```python
from build123d import *

# Parameters (mm, degrees)
F0_W     = 12.8
F0_H     = 6.4
F1_DEPTH = 1
F0_W_2   = 20
F0_H_2   = 12
F2_DEPTH = 160
F3_R     = 5
F4_T     = -2
F5_DEPTH = 2


with BuildPart() as f1:
    # F0 (on Top) → F1 (new body)
    with BuildSketch(Plane.XY):
        Rectangle(F0_W, F0_H)
    extrude(amount=-F1_DEPTH)

    # F0 (on Top) → F2 (join)
    with BuildSketch(Plane.XY):
        Rectangle(F0_W_2, F0_H_2)
        Rectangle(F0_W, F0_H, mode=Mode.SUBTRACT)
        Rectangle(F0_W, F0_H)
    extrude(amount=F2_DEPTH)

    # F3
    f3_edges = [f1.edges().sort_by_distance(p)[0] for p in [
        (-10, -6, 80),
        (10, -6, 80),
        (10, 6, 80),
        (-10, 6, 80),
    ]]
    fillet(f3_edges, radius=F3_R)

    # F4
    f4_openings = [f1.faces().sort_by_distance(p)[0] for p in [
        (0, 0, 160),
    ]]
    offset(amount=F4_T, openings=f4_openings, kind=Kind.INTERSECTION)

    # F5 (add): a face of the model
    f5_faces = [f1.faces().sort_by_distance(p)[0] for p in [
        (0, 0, 1),
    ]]
    extrude(f5_faces, amount=F5_DEPTH)


solid = f1.part
```
CAD build for the part. Positions are in the model's coordinates, mm. A direction names the side the tool comes from. Coordinates: 2 decimals unless noted, no trailing zeros. Order: outer loops, then holes, each group sorted by start corner. A loop starts at its lowest first (then second) coordinate and runs counter-clockwise, first axis right, second up. Notation, with made-up numbers: (-26.5, 73.25) - (22.5, 73.25) arc R16 cw to (22.5, 82.25) - close; hole circle Ø6 at (58, 63). An arc over 180 degrees is marked (long way). Answer in a Markdown table with one row per item.
1. Pull direction X, two halves, no side cores. Call faces 1 (the face through (7.1, -3.14, 82.11)), 2 (the face through (8, 5, 81)), 3 (the face through (-9, 4, 81)): +X half, -X half, draft (parallel to the pull), parting line (faces both ways), or undercut.
Answer:
| item | result |
|---|---|
| face 1 | undercut |
| face 2 | +X half |
| face 3 | -X half |
2. Slice it at A-A, the plane z = 21. List the corners of the cut face in (x, y).
Answer:
| item | result |
|---|---|
| outline | (-10, -1) arc R5 ccw to (-5, -6) - (5, -6) arc R5 ccw to (10, -1) - (10, 1) arc R5 ccw to (5, 6) - (-5, 6) arc R5 ccw to (-10, 1) - close; hole (-8, -1) arc R3 ccw to (-5, -4) - (5, -4) arc R3 ccw to (8, -1) - (8, 1) arc R3 ccw to (5, 4) - (-5, 4) arc R3 ccw to (-8, 1) - close |
3. Flat gauge pins, fed straight in: P1, Ø1.5, axis at y = -3, z = 19, coming from the +X side; P2, Ø0.5, axis at x = -2, z = -0.5, coming from the +Y side; P3, Ø1.5, axis at x = 2, y = -4.5, coming from the -Z side; P4, Ø1, axis at y = -1.5, z = 25.5, coming from the -X side. Where does each tip first touch, or does it go through?
Answer:
| item | result |
|---|---|
| P1 | x = 9.84 |
| P2 | y = 3.2 |
| P3 | z = 0 |
| P4 | x = -10 |
4. Drill centre lines: L1, parallel to Y at x = 2.5, z = 34.5; L2, parallel to Z at x = 0.75, y = -0.25; L3, parallel to Z at x = -3, y = -3.5. Where is each one in solid material? Low to high. Write a range as from..to.
Answer:
| item | result |
|---|---|
| L1 | -6..-4, 4..6 |
| L2 | -1..3 |
| L3 | 0..2 |
5. 3-axis set-ups, long thin cutter, end or side, ignore diameter. For faces 4 (the face through (0, 0, -1)), 5 (the face through (-7.14, 3.1, 82.11)): which of +Z, -Z, +X, -X, +Y, -Y reach the whole face in a straight line?
Answer:
| item | result |
|---|---|
| face 4 | -Z, +X, -X, +Y, -Y |
| face 5 | +Z |
6. Slice it at B-B, the plane x = 2.75. List the corners of the cut face in (y, z), then the cut area to 3 significant figures.
Answer:
| item | result |
|---|---|
| outline | (-6, 0) - (-3.2, 0) - (-3.2, -1) - (3.2, -1) - (3.2, 0) - (6, 0) - (6, 160) - (4, 160) - (4, 2) - (1.2, 2) - (1.2, 3) - (-1.2, 3) - (-1.2, 2) - (-4, 2) - (-4, 160) - (-6, 160) - close |
| area | 665 mm² |
